from build123d import *

# Parameters (mm, degrees)
SKETCH035_R     = 15
PAD013_DEPTH    = 5.3
SKETCH036_R     = 9
POCKET019_DEPTH = 1
SKETCH037_R     = 1.65
POCKET020_DEPTH = 5
FILLET008_R     = 1
CHAMFER003_SIZE = 1


with BuildPart() as part:
    # Sketch035 → Pad013 (new body)
    with BuildSketch(Plane.XY):
        Circle(SKETCH035_R)
    extrude(amount=PAD013_DEPTH)

    # Sketch036 → Pocket019 (cut)
    with BuildSketch(Plane.XY.offset(5.3)):
        Circle(SKETCH036_R)
    extrude(amount=-POCKET019_DEPTH, mode=Mode.SUBTRACT)

    # Sketch037 (on Face5 of Pocket019) → Pocket020 (cut)
    with BuildSketch(Plane.XY.offset(4.3)):
        Circle(SKETCH037_R)
    extrude(amount=-POCKET020_DEPTH, mode=Mode.SUBTRACT)

    # Fillet008
    fillet008_edges = [part.edges().sort_by_distance(p)[0] for p in [
        (-15, 0, 5.3),
    ]]
    fillet(fillet008_edges, radius=FILLET008_R)

    # Chamfer003
    chamfer003_edges = [part.edges().sort_by_distance(p)[0] for p in [
        (-1.65, 0, 4.3),
    ]]
    chamfer(chamfer003_edges, length=CHAMFER003_SIZE)


with BuildPart() as part_1:
    # Body009 placement: moved
    add(part.part.moved(Location((59.5, 37.5, 85))))


solid = part_1.part
Model file for the job. Use its own axes, mm. A direction names the side the tool comes from. Round coordinates to 2 decimals unless told otherwise and drop trailing zeros. Order: outer loops, then holes, each group sorted by start corner. A loop starts at its lowest first (then second) coordinate and runs counter-clockwise, first axis right, second up.
(1) Pin check, flat tips, straight feed: pin 1 (1 mm diameter, centred on x = 48.5, z = 88.5, fed in from +Y); pin 2 (11 mm diameter, centred on x = 59.5, y = 37.5, fed in from +Z); pin 3 (1 mm diameter, centred on y = 30.5, z = 86, fed in from -X). Stop position of each tip, or through.
(2) Band-saw the part on C-C (z = 87). List the corners of the cut face in (x, y).
(3) Band-saw the part on A-A (x = 59.5). List the corners of the cut face in (y, z).
(4) Drill centre lines: line 1 (Y direction, x = 59.5, z = 87); line 2 (Z direction, x = 68, y = 38.25); line 3 (X direction, y = 39.25, z = 89.35). Where is each one in solid material? Low to high.
(5) 3-axis set-ups, long thin cutter, end or side, ignore diameter. For faces 1 (the face through (57.85, 37.57, 86.67)), 2 (the face through (57, 36, 89.3)): which of +Z, -Z, +X, -X, +Y, -Y reach the whole face in a straight line?
(6) Band-saw the part on B-B (y = 37.5). List the corners of the cut face in (x, z), then the cut area to 3 significant figures.
(7) Band-saw the part on D-D (z = 88.8). List the corners of the cut face in (x, y).
(8) Pull direction Y, two halves, no side cores. Call faces 3 (the face through (64.34, 45.09, 89.81)), 4 (the face through (69, 38, 90.3)), 5 (the face through (48.444, 47.638, 87.12)): released by +Y, released by -Y, zero draft, split by the parting line, or undercut.
Verdict:
1. pin 1: stops at y = 48.21
1. pin 2: stops at z = 89.3
1. pin 3: stops at x = 45.98
2. outline: circle Ø30 at (59.5, 37.5); hole circle Ø3.3 at (59.5, 37.5)
3. outline: (22.5, 85) - (35.85, 85) - (35.85, 88.3) - (34.85, 89.3) - (28.5, 89.3) - (28.5, 90.3) - (23.5, 90.3) arc R1 ccw to (22.5, 89.3) - close; (39.15, 85) - (52.5, 85) - (52.5, 89.3) arc R1 ccw to (51.5, 90.3) - (46.5, 90.3) - (46.5, 89.3) - (40.15, 89.3) - (39.15, 88.3) - close
4. line 1: y = 22.5 to 35.85, 39.15 to 52.5
4. line 2: z = 85 to 89.3
4. line 3: x = 44.6 to 50.67, 68.33 to 74.4
5. face 1: +Z, -Z
5. face 2: +Z
6. outline: (44.5, 85) - (57.85, 85) - (57.85, 88.3) - (56.85, 89.3) - (50.5, 89.3) - (50.5, 90.3) - (45.5, 90.3) arc R1 ccw to (44.5, 89.3) - close; (61.15, 85) - (74.5, 85) - (74.5, 89.3) arc R1 ccw to (73.5, 90.3) - (68.5, 90.3) - (68.5, 89.3) - (62.15, 89.3) - (61.15, 88.3) - close
6. area: 125 mm2
7. outline: circle Ø30 at (59.5, 37.5); hole circle Ø4.3 at (59.5, 37.5)
8. face 3: undercut
8. face 4: zero draft
8. face 5: split by the parting line
